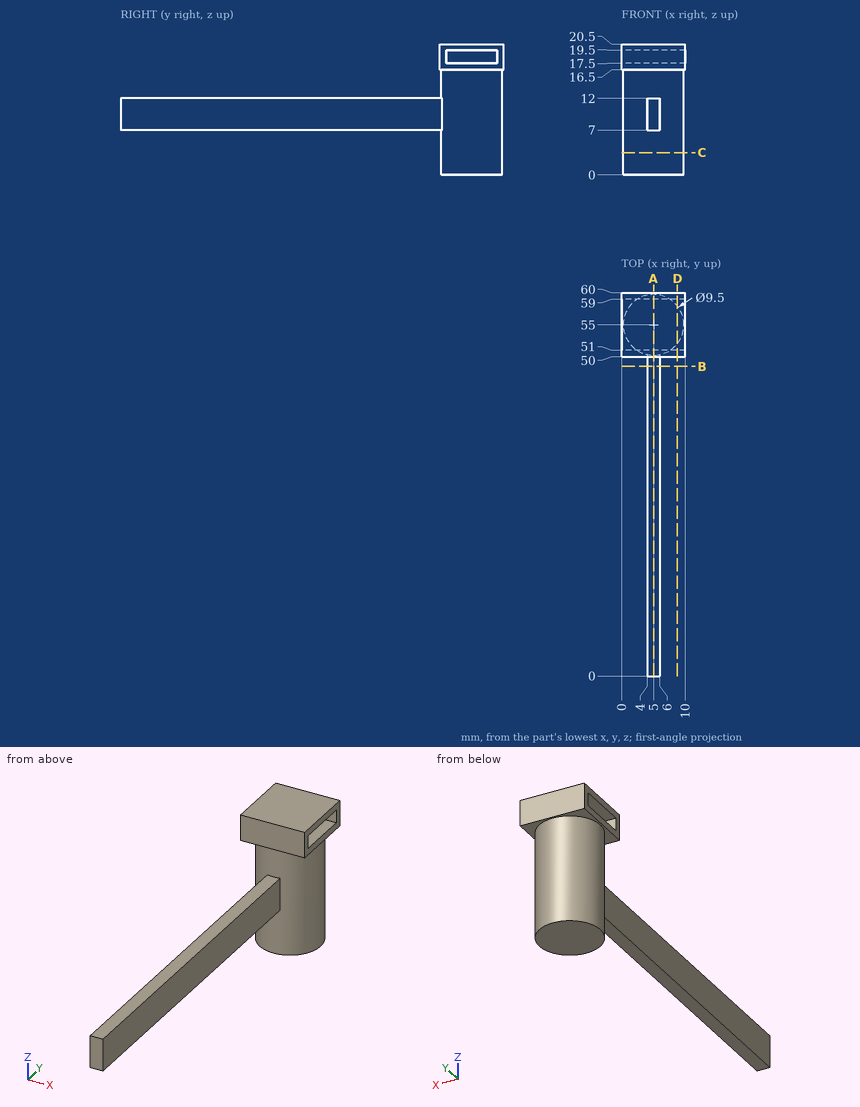
Drawing for the job (mm, zero at the part's lowest x, y, z). Give positions to 0.01 mm unless a question says otherwise; leave off trailing zeros. Order: outer loops, then holes, each group sorted by start corner. A loop starts at its lowest first (then second) coordinate and runs counter-clockwise, first axis right, second up. Notation, with made-up numbers: (20.5, 59) -> (52.5, 59) arc R20 ccw to (52.5, 85) -> close; hole circle Ø11 at (23, -2). An arc over 180 degrees is marked (long way). Use one line per item in the form item = value.
(1) Saw through at A-A (x = 5). Write the cut outline in (y, z).
Solution:
outline = (0, 7) -> (50.25, 7) -> (50.25, 0) -> (59.75, 0) -> (59.75, 16.5) -> (60, 16.5) -> (60, 20.5) -> (50, 20.5) -> (50, 16.5) -> (50.25, 16.5) -> (50.25, 12) -> (0, 12) -> close; hole (51, 17.5) -> (59, 17.5) -> (59, 19.5) -> (51, 19.5) -> close
(2) Saw through at B-B (y = 48.5). Write the cut outline in (x, z).
Solution:
outline = (4, 7) -> (6, 7) -> (6, 12) -> (4, 12) -> close
(3) Saw through at C-C (z = 3.5). Write the cut outline in (x, y).
Solution:
outline = circle Ø9.5 at (5, 55)
(4) Flat gauge pins, fed straight in: P1, Ø4, axis at x = 4, z = 6, coming from the +Y side; P2, Ø4, axis at y = 7.5, z = 5.5, coming from the +X side; P3, Ø1, axis at x = 5, y = 15, coming from the +Z side; P4, Ø3, axis at x = 2, y = 34.5, coming from the -Z side. Where does each tip first touch, or does it go through?
Solution:
P1 = 59.75
P2 = 6
P3 = 12
P4 = through
(5) Saw through at D-D (x = 8.75). Write the cut outline in (y, z).
Solution:
outline = (50, 16.5) -> (52.08, 16.5) -> (52.08, 0) -> (57.92, 0) -> (57.92, 16.5) -> (60, 16.5) -> (60, 20.5) -> (50, 20.5) -> close; hole (51, 17.5) -> (59, 17.5) -> (59, 19.5) -> (51, 19.5) -> close
(6) Drill centre lines: line 1 (Z direction, x = 9, y = 51.5); line 2 (Y direction, x = 7.5, z = 19); line 3 (Y direction, x = 4.75, z = 14.75). Where is each one in solid material? Low to high. Write a range as from..to.
Solution:
line_1 = 16.5..17.5, 19.5..20.5
line_2 = 50..51, 59..60
line_3 = 50.26..59.74
